Autodesk Inventor part; units mm, degrees
ref_plane "YZ Plane" through (0, 0, 0) normal (1, 0, 0) x (0, 1, 0)
ref_plane "XZ Plane" through (0, 0, 0) normal (0, 1, 0) x (-1, 0, 0)
ref_plane "XY Plane" through (0, 0, 0) normal (0, 0, 1) x (1, 0, 0)
sketch "Boceto1" plane through (0, 0, 0) normal (0, 0, 1) x (1, 0, 0)
  circle A0 centre (0, 0) radius 2
  circle A1 centre (0, 0) radius 3.25
  dimension "d0" = 4
  dimension "d1" = 6.5
extrude "Extrusión1" add sketch "Boceto1" along normal blind 20 contours A0
extrude "Extrusión2" add sketch "Boceto1" against normal blind 4 contours A0 | A1
sketch "Boceto2" plane through (0, 0, -4) normal (0, 0, -1) x (-1, 0, 0)
  line L0 (2, 0) -> (1, -1.7321)
  line L1 (1, -1.7321) -> (-1, -1.7321)
  line L2 (-1, -1.7321) -> (-2, 0)
  line L3 (-2, 0) -> (-1, 1.7321)
  line L4 (-1, 1.7321) -> (1, 1.7321)
  line L5 (1, 1.7321) -> (2, 0)
  point P0 (0, 0)
  point P1 (0, 0)
  dimension "d6" = 4
extrude "Extrusión3" cut sketch "Boceto2" against normal blind 2
thread "Rosca1"
properties part number "TornilloM4X20mm" material "Acero inoxidable"
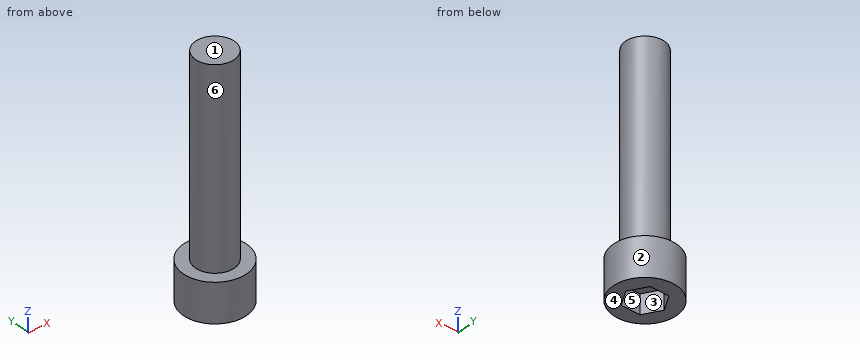
Geometry: final body of the model. Coordinates: model frame, mm. Face numbers are marked on the shaded views. A direction names the side the tool comes from. Give positions to 0.01 mm unless a question says otherwise; leave off trailing zeros. Order: outer loops, then holes, each group sorted by start corner. A loop starts at its lowest first (then second) coordinate and runs counter-clockwise, first axis right, second up. Notation, with made-up numbers: (-13, 88.25) -> (24, 88.25) arc R22 cw to (24, 95.25) -> close; hole circle Ø7 at (32.5, 31). An arc over 180 degrees is marked (long way). Put each result on its own line as item: value.
Q1. Section A-A, the plane x = 0. Return loops of the section in (y, z), then the cut area to 3 significant figures.
Here are the results:
outline: (-3.25, -4) -> (-1.73, -4) -> (-1.73, -2) -> (1.73, -2) -> (1.73, -4) -> (3.25, -4) -> (3.25, 0) -> (2, 0) -> (2, 20) -> (-2, 20) -> (-2, 0) -> (-3.25, 0) -> close
area: 99.1 mm^2
Q2. Section D-D, the plane z = -1.5. Return loops of the section in (x, y).
Here are the results:
outline: circle Ø6.5 at (0, 0)
Q3. Material intervals for L1, parallel to Z at x = 2.5, y = -0.75; L2, parallel to Z at x = -0.75, y = 1; L3, parallel to Y at x = -1, z = 1, sorted ascending.
Here are the results:
L1: z = -4 to 0
L2: z = -2 to 20
L3: y = -1.73 to 1.73
Q4. Pin query (flat end, axial travel): pin 1 (1 mm diameter, centred on x = -2, z = 2, fed in from -Y); pin 2 (1.5 mm diameter, centred on y = 1, z = 10.5, fed in from -X); pin 3 (1 mm diameter, centred on x = 0.5, y = -0.5, fed in from -Z). Return the tip coordinate at first contact, or that it passes through.
Here are the results:
pin 1: stops at y = -1.32
pin 2: stops at x = -1.98
pin 3: stops at z = -2
Q5. Section B-B, the plane z = 13. Return loops of the section in (x, y), then the cut area to 3 significant figures.
Here are the results:
outline: circle Ø4 at (0, 0)
area: 12.6 mm^2
Q6. Reachability of the marked faces 4, 5 and 6 from +Z, -Z, +X, -X, +Y, -Y: full face, straight path, thin tool, end or side. Return the list, or none.
Here are the results:
face 4: -Z, +X, -X, +Y, -Y
face 5: -Z
face 6: +Z
Q7. Draft query along X for the marked faces 1, 2 and 3. Return one class per face: released by +X, released by -X, zero draft, split by the parting line, or undercut.
Here are the results:
face 1: zero draft
face 2: split by the parting line
face 3: undercut
Q8. Section C-C, the plane y = -1.25. Return loops of the section in (x, z), then the cut area to 3 significant figures.
Here are the results:
outline: (-3, -4) -> (-1.28, -4) -> (-1.28, -2) -> (1.28, -2) -> (1.28, -4) -> (3, -4) -> (3, 0) -> (1.56, 0) -> (1.56, 20) -> (-1.56, 20) -> (-1.56, 0) -> (-3, 0) -> close
area: 81.3 mm^2
